from build123d import *

# Parameters (mm, degrees)
F0_R      = 1
F1_DEPTH  = 8
F2_R      = 2.75
F3_DEPTH  = 80
F4_SIZE2  = 1
F4_SIZE   = 4
F5_R      = 6
F5_R_2    = 2.75
F6_DEPTH  = 5
F7_DEPTH  = 10
F12_R     = 2.75
F12_R_2   = 1.5
F13_DEPTH = 55
F15_D     = 4.2
F16_W     = 4
F16_H     = 15
F17_DEPTH = 2.5
F24_DEPTH = 15


with BuildPart() as f1:
    # F0 (on Front) → F1 (new body)
    with BuildSketch(Plane.XZ):
        Circle(F0_R)
    extrude(amount=-F1_DEPTH)

    # F2 (on face) → F3 (join)
    with BuildSketch(Plane.XZ):
        Circle(F2_R)
    extrude(amount=F3_DEPTH)

    # F4
    f4_edges = [f1.edges().sort_by_distance(p)[0] for p in [
        (-2.75, 0, 0),
    ]]
    f4_side = f1.faces().sort_by_distance((-2.75, -40, 0))[0]
    chamfer(f4_edges, length=F4_SIZE, length2=F4_SIZE2, reference=f4_side)

    # F5 (on face) → F6 (join)
    with BuildSketch(Plane.XZ.offset(80)):
        Circle(F5_R)
        Circle(F5_R_2, mode=Mode.SUBTRACT)
    extrude(amount=-F6_DEPTH)

    # F7 (add): a face of the model
    f7_faces = [f1.faces().sort_by_distance(p)[0] for p in [
        (0, -80, 0),
    ]]
    extrude(f7_faces, amount=F7_DEPTH)

    # F12 (on face) → F13 (cut)
    with BuildSketch(Plane(origin=(0, -75, 0), x_dir=(-1, 0, 0), z_dir=(0, 1, 0))):
        Circle(F12_R)
        Circle(F12_R_2, mode=Mode.SUBTRACT)
    extrude(amount=F13_DEPTH, mode=Mode.SUBTRACT)

    # F15 (through all)
    with Locations(Plane.YZ.offset(6)):
        with Locations((-86, 0)):
            Hole(F15_D / 2)

    # F16 (on offset) → F17 (cut)
    with BuildSketch(Plane.XY.offset(6)):
        with Locations((0, -82.5)):
            Rectangle(F16_W, F16_H)
    extrude(amount=-F17_DEPTH, mode=Mode.SUBTRACT)

    # F23 (on face) → F24 (cut)
    with BuildSketch(Plane.XZ.offset(90)):
        with BuildLine():
            ThreePointArc((-3.1795155854, 5.0882885769), (-5.7529184092, 1.7040920682), (-5.4378467222, -2.5357095704))
            Line((-5.4378467222, -2.5357095704), (-4.5315389352, -2.1130913087))
            ThreePointArc((-4.5315389352, -2.1130913087), (-4.7940986743, 1.4200767235), (-2.6495963212, 4.2402404808))
            Line((-2.6495963212, 4.2402404808), (-3.1795155854, 5.0882885769))
        make_face()
    extrude(amount=-F24_DEPTH, mode=Mode.SUBTRACT)


solid = f1.part
The model under review builds one solid part; all positions refer to its coordinate system, in mm. A direction names the side the tool comes from. Coordinates: 2 decimals unless noted, no trailing zeros. Loops run counter-clockwise (first coordinate to the right, second up) from the corner with the lowest first, then second, coordinate; pieces in that order, holes last. Notation, with made-up numbers: (63.25, -33) -> (105.25, -33) arc R21 cw to (105.25, 3) -> close; hole circle Ø5 at (41, 31). An arc over 180 degrees is marked (long way). Use a Markdown table: item, result. Add a question column.
1. Clearance check with flat-ended pins moving along their axes: pin 1 Ø1.1 at (y, z) = (-82, 4.5) entering from -X; pin 2 Ø6 at (x, y) = (2.5, -63) entering from -Z; pin 3 Ø5 at (y, z) = (-55.5, 1) entering from +X; pin 4 Ø5.5 at (x, z) = (-1, 2.5) entering from +Y. State where each tip first meets the part, or that it passes through.
2. Machinability: for faces 1 (the face through (2, -83, 5)), 2 (the face through (1.5, -47.89, 0.07)), 3 (the face through (0, 4, -1)), which of the approach directions +Z, -Z, +X, -X, +Y, -Y give a long, thin tool a straight path to every point of the face, cutting with its end or side? Answer none if there is none.
3. Draft analysis for pull direction Y (two halves, no side actions). For faces 4 (the face through (0.42, -83.9, 0.09)), 5 (the face through (0, -90, 0)), 6 (the face through (-0.462, -1.528, -2.081)), state which applies: pulls with the +Y half, pulls with the -Y half, needs draft (parallel to the pull), parting line crosses it, or undercut.
4. Add section D-D on y = -61. Write out the cut boundary in (x, z).
5. To check wall thickness, follow line 1 (Y direction, x = 3, z = 0); line 2 (Y direction, x = -1, z = -4.25); line 3 (Y direction, x = 0, z = 0). State the ranges of each line that lie inside material, in increasing order.
6. Add section B-B on z = 0. Write out the cut boundary in (x, y), plus the area to 3 significant figures.
7. Add section A-A on x = 0. Write out the cut boundary in (y, z), plus the area to 3 significant figures.
Returned:
| question | item | result |
|---|---|---|
| 1 | pin 1 | stops at x = -3.16 |
| 1 | pin 2 | stops at z = -1.5 |
| 1 | pin 3 | stops at x = 1.5 |
| 1 | pin 4 | stops at y = 8 |
| 2 | face 1 | +Z, +Y, -Y |
| 2 | face 2 | none |
| 2 | face 3 | +Y |
| 3 | face 4 | undercut |
| 3 | face 5 | pulls with the -Y half |
| 3 | face 6 | pulls with the +Y half |
| 4 | outline | circle Ø3 at (0, 0) |
| 5 | line 1 | y = -90 to -88.1, -83.9 to -75 |
| 5 | line 2 | y = -90 to -75 |
| 5 | line 3 | y = -90 to -88.1, -83.9 to 8 |
| 6 | outline | (-5, -90) -> (6, -90) -> (6, -88.1) -> (-5, -88.1) -> close; (-5, -83.9) -> (6, -83.9) -> (6, -75) -> (1.5, -75) -> (1.5, -20) -> (2.75, -20) -> (2.75, -4) -> (1.75, 0) -> (1, 0) -> (1, 8) -> (-1, 8) -> (-1, 0) -> (-1.75, 0) -> (-2.75, -4) -> (-2.75, -20) -> (-1.5, -20) -> (-1.5, -75) -> (-5, -75) -> close |
| 6 | area | 406 mm² |
| 7 | outline | (-90, -6) -> (-75, -6) -> (-75, -1.5) -> (-20, -1.5) -> (-20, -2.75) -> (-4, -2.75) -> (0, -1.75) -> (0, -1) -> (8, -1) -> (8, 1) -> (0, 1) -> (0, 1.75) -> (-4, 2.75) -> (-20, 2.75) -> (-20, 1.5) -> (-75, 1.5) -> (-75, 3.5) -> (-90, 3.5) -> close; hole circle Ø4.2 at (-86, 0) |
| 7 | area | 416 mm² |
